Solid Edge part; units mm, degrees
sketch "Sketch1" plane through (0, 0, 0) normal (0, 0, 1) x (1, 0, 0)
  circle A0 centre (0, 0) radius 1.5
extrude "Protrusion1" add sketch "Sketch1" along normal blind 6.5
sketch "Sketch2" plane through (0, 0, 6.5) normal (0, 0, 1) x (1, 0, 0)
  circle A0 centre (0, 0) radius 2.5
extrude "Head" add sketch "Sketch2" along normal blind 1
fillet "Round___Head" radius 0.5 1 edges at (-2.5, 0, 7.5)
sketch "Sketch3" plane through (0, 0, 7.5) normal (0, 0, 1) x (1, 0, 0)
  line L0 (-0.5, -2.4495) -> (-0.5, 2.4495)
  line L1 (0.5, 2.4495) -> (0.5, -2.4495)
  arc A0 (0.5, -2.4495) -> (-0.5, -2.4495) centre (0, 0) cw
  arc A1 (-0.5, 2.4495) -> (0.5, 2.4495) centre (0, 0) cw
extrude "Cutout___Head" cut sketch "Sketch3" against normal blind 0.5
cosmetic_thread "Thread1"
properties material "Stainless Steel, 420"
Source: CAD feature listing. Evaluate the final solid. Frame: model axes, mm. A direction names the side the tool comes from. Coordinates: 2 decimals unless noted, no trailing zeros. Write each loop counter-clockwise with the first axis right and the second up, starting at its lowest first coordinate (ties: lowest second). Pieces come first, ordered by that corner, then holes. Notation, with made-up numbers: M 36.25,20.5 L 53.25,20.5 A15 ccw 53.25,45.5 Z; hole C 48.5,59.5 d7. An arc over 180 degrees is marked long. Use a Markdown table: item, result.
1) Section A-A, the plane y = 0. Output: boundary loops of the cut face in (x, z), then the cut area to 3 significant figures.
Conclusion:
| item | result |
|---|---|
| outline | M -2.5,6.5 L -1.5,6.5 L -1.5,0 L 1.5,0 L 1.5,6.5 L 2.5,6.5 L 2.5,7 A0.5 ccw 2,7.5 L 0.5,7.5 L 0.5,7 L -0.5,7 L -0.5,7.5 L -2,7.5 A0.5 ccw -2.5,7 Z |
| area | 23.9 mm^2 |
2) Section B-B, the plane x = 0. Output: boundary loops of the cut face in (y, z).
Conclusion:
| item | result |
|---|---|
| outline | M -2.5,6.5 L -1.5,6.5 L -1.5,0 L 1.5,0 L 1.5,6.5 L 2.5,6.5 L 2.5,7 L -2.5,7 Z |
3) Reachability of faces 4 (the flat face through (2, 0, 6.5)), 5 (the flat face through (1, 0, 7.5)) from +Z, -Z, +X, -X, +Y, -Y: full face, straight path, thin tool, end or side. Return the list, or none.
Conclusion:
| item | result |
|---|---|
| face 4 | -Z |
| face 5 | +Z, +X, -X, +Y, -Y |
4) Ray query, L1, parallel to Z at x = -1.55, y = -0.65; L2, parallel to Z at x = 0.4, y = -0.2; L3, parallel to Y at x = -0.9, z = 0.5. Return the intervals inside material, ascending.
Conclusion:
| item | result |
|---|---|
| L1 | z = 6.5 to 7.5 |
| L2 | z = 0 to 7 |
| L3 | y = -1.2 to 1.2 |
5) Section C-C, the plane z = 7.25. Output: boundary loops of the cut face in (x, y), then the cut area to 3 significant figures.
Conclusion:
| item | result |
|---|---|
| outline | M -0.5,-2.38 L -0.5,2.38 A2.43 ccw Z; M 0.5,-2.38 A2.43 ccw 0.5,2.38 Z |
| area | 13.8 mm^2 |
6) First-contact query: pin 1 Ø0.8 at (x, y) = (0, 1) entering from +Z; pin 2 Ø1 at (x, z) = (-1.5, 3.5) entering from +Y; pin 3 Ø2 at (x, z) = (1, 5) entering from -Y. Flat tips, straight axial feed; report the tip coordinate or a pass-through.
Conclusion:
| item | result |
|---|---|
| pin 1 | stops at z = 7 |
| pin 2 | stops at y = 1.12 |
| pin 3 | stops at y = -1.5 |
7) Mould query, pull axis X, two halves, no side actions, for faces 1 (the flat face through (0, 0, 0)), 2 (the flat face through (0, 0, 7)), 3 (the cylindrical face through (-0.54, 2.44, 6.75)). Classes: pulls with the +X half, pulls with the -X half, needs draft (parallel to the pull), parting line crosses it, or undercut.
Conclusion:
| item | result |
|---|---|
| face 1 | needs draft |
| face 2 | undercut |
| face 3 | parting line crosses it |
8) Section D-D, the plane z = 1. Output: boundary loops of the cut face in (x, y), then the cut area to 3 significant figures.
Conclusion:
| item | result |
|---|---|
| outline | C 0,0 d3 |
| area | 7.07 mm^2 |
